from build123d import *

# Parameters (mm, degrees)
F1_DEPTH = 9.5
F2_W     = 116.8
F2_H     = 3
F3_DEPTH = 30
F4_R     = 1.5
F5_DEPTH = 25


with BuildPart() as f1:
    # F0 (on Top) → F1 (new body)
    with BuildSketch(Plane.XY):
        Polygon((0, 0), (-24.4, 0), (-36.4, 0), (-52.4, 0), (-52.4, -3), (-36.4, -3), (-36.4, -7.5), (-24.4, -7.5), (-24.4, -4.5), (-33.4, -4.5), (-33.4, -3), (-24.4, -3), (0, -3), align=None)
        Polygon((36.4, 0), (0, 0), (0, -3), (36.4, -3), (36.4, -7.5), (48.4, -7.5), (48.4, -4.5), (39.4, -4.5), (39.4, -3), (48.4, -3), (64.4, -3), (64.4, 0), (48.4, 0), align=None)
    extrude(amount=F1_DEPTH)

    # F2 (on face) → F3 (join)
    with BuildSketch(Plane(origin=(0, 0, 0), x_dir=(1, 0, 0), z_dir=(0, 0, -1))):
        with Locations((6, 1.5)):
            Rectangle(F2_W, F2_H)
    extrude(amount=-F3_DEPTH)

    # F4 (on face) → F5 (cut)
    with BuildSketch(Plane(origin=(0, 0, 0), x_dir=(-1, 0, 0), z_dir=(0, 1, 0))):
        with Locations((47.4, 25)):
            Circle(F4_R)
        with Locations((-59.4, 25)):
            Circle(F4_R)
        with Locations((-59.4, 5)):
            Circle(F4_R)
        with Locations((47.4, 5)):
            Circle(F4_R)
        with Locations((-6, 25)):
            Circle(F4_R)
        with Locations((-6, 5)):
            Circle(F4_R)
    extrude(amount=-F5_DEPTH, mode=Mode.SUBTRACT)


solid = f1.part
Source: CAD feature listing. Evaluate the final solid. Frame: model axes, mm. A direction names the side the tool comes from. Give positions to 0.01 mm unless a question says otherwise; leave off trailing zeros. Loops run counter-clockwise (first coordinate to the right, second up) from the corner with the lowest first, then second, coordinate; pieces in that order, holes last. Notation, with made-up numbers: (30, -2) -> (57, -2) arc R32 ccw to (57, 29) -> close; hole circle Ø7 at (40, 66.25). An arc over 180 degrees is marked (long way). Use a Markdown table: item, result. Add a question column.
1) Section query A-A, the plane x = 59.4. Return the cut outline in (y, z).
2) Pull-direction query (X, two-part tool) for faces 1 (the face through (48.4, -6, 5)), 2 (the face through (5, -2, 30)), 3 (the face through (-48.83, -1.48, 5.45)); classes: +X half, -X half, draft (parallel to the pull), parting line (faces both ways), or undercut.
3) Line query: line 1 along Z through (x, y) = (59.4, -0.7); line 2 along X through (y, z) = (-0.5, 6.25); line 3 along Y through (x, z) = (57, 21). Output: solid intervals per line, ascending. Write a range as [from, to].
4) Reachability of faces 4 (the face through (-24.4, -6, 5)), 5 (the face through (5, -2, 0)), 6 (the face through (42, -6, 9.5)), 7 (the face through (44, -4.5, 5)), 8 (the face through (-36.4, -5, 5)) from +Z, -Z, +X, -X, +Y, -Y: full face, straight path, thin tool, end or side. Return the list, or none.
5) First-contact query: pin 1 (3.5 mm diameter, centred on x = -29, y = -6.5, fed in from +Z); pin 2 (2 mm diameter, centred on y = -6, z = 4, fed in from -X); pin 3 (1.5 mm diameter, centred on y = -6.5, z = 7, fed in from +X). Flat tips, straight axial feed; report the tip coordinate or a pass-through.
6) Section query C-C, the plane y = -5.5. Return the cut outline in (x, z), then the cut area to 3 significant figures.
7) Section query D-D, the plane z = 25. Return the cut outline in (x, y), then the cut area to 3 significant figures.
8) Section query B-B, the plane z = 5. Return the cut outline in (x, y), then the cut area to 3 significant figures.
Numbers:
| question | item | result |
|---|---|---|
| 1 | outline | (-3, 0) -> (0, 0) -> (0, 3.5) -> (-3, 3.5) -> close; (-3, 6.5) -> (0, 6.5) -> (0, 23.5) -> (-3, 23.5) -> close; (-3, 26.5) -> (0, 26.5) -> (0, 30) -> (-3, 30) -> close |
| 2 | face 1 | +X half |
| 2 | face 2 | draft |
| 2 | face 3 | undercut |
| 3 | line 1 | z = [0, 3.5], [6.5, 23.5], [26.5, 30] |
| 3 | line 2 | x = [-52.4, -48.23], [-46.57, 5.17], [6.83, 58.57], [60.23, 64.4] |
| 3 | line 3 | y = [-3, 0] |
| 4 | face 4 | +Z, -Z, -Y |
| 4 | face 5 | -Z, +X, -X, +Y, -Y |
| 4 | face 6 | +Z, +X, -X, -Y |
| 4 | face 7 | +Z, -Z, +X |
| 4 | face 8 | +Z, -Z, -X, -Y |
| 5 | pin 1 | stops at z = 9.5 |
| 5 | pin 2 | stops at x = -36.4 |
| 5 | pin 3 | stops at x = 48.4 |
| 6 | outline | (-36.4, 0) -> (-24.4, 0) -> (-24.4, 9.5) -> (-36.4, 9.5) -> close; (36.4, 0) -> (48.4, 0) -> (48.4, 9.5) -> (36.4, 9.5) -> close |
| 6 | area | 228 mm2 |
| 7 | outline | (-52.4, -3) -> (-48.9, -3) -> (-48.9, 0) -> (-52.4, 0) -> close; (-45.9, -3) -> (4.5, -3) -> (4.5, 0) -> (-45.9, 0) -> close; (7.5, -3) -> (57.9, -3) -> (57.9, 0) -> (7.5, 0) -> close; (60.9, -3) -> (64.4, -3) -> (64.4, 0) -> (60.9, 0) -> close |
| 7 | area | 323 mm2 |
| 8 | outline | (-52.4, -3) -> (-48.9, -3) -> (-48.9, 0) -> (-52.4, 0) -> close; (-45.9, -3) -> (-36.4, -3) -> (-36.4, -7.5) -> (-24.4, -7.5) -> (-24.4, -4.5) -> (-33.4, -4.5) -> (-33.4, -3) -> (4.5, -3) -> (4.5, 0) -> (-45.9, 0) -> close; (7.5, -3) -> (36.4, -3) -> (36.4, -7.5) -> (48.4, -7.5) -> (48.4, -4.5) -> (39.4, -4.5) -> (39.4, -3) -> (57.9, -3) -> (57.9, 0) -> (7.5, 0) -> close; (60.9, -3) -> (64.4, -3) -> (64.4, 0) -> (60.9, 0) -> close |
| 8 | area | 404 mm2 |
